Source: three-view drawing plus pictorial views. Frame: mm from the lowest corner of the part. A direction names the side the tool comes from. Give positions to 0.01 mm unless a question says otherwise; leave off trailing zeros. Order: outer loops, then holes, each group sorted by start corner. A loop starts at its lowest first (then second) coordinate and runs counter-clockwise, first axis right, second up. Notation, with made-up numbers: M 31,38 L 44,38 A32 ccw 44,74 Z; hole C 51,61.25 d7. An arc over 180 degrees is marked long. One line per item, written item: value. Start each with the question number.
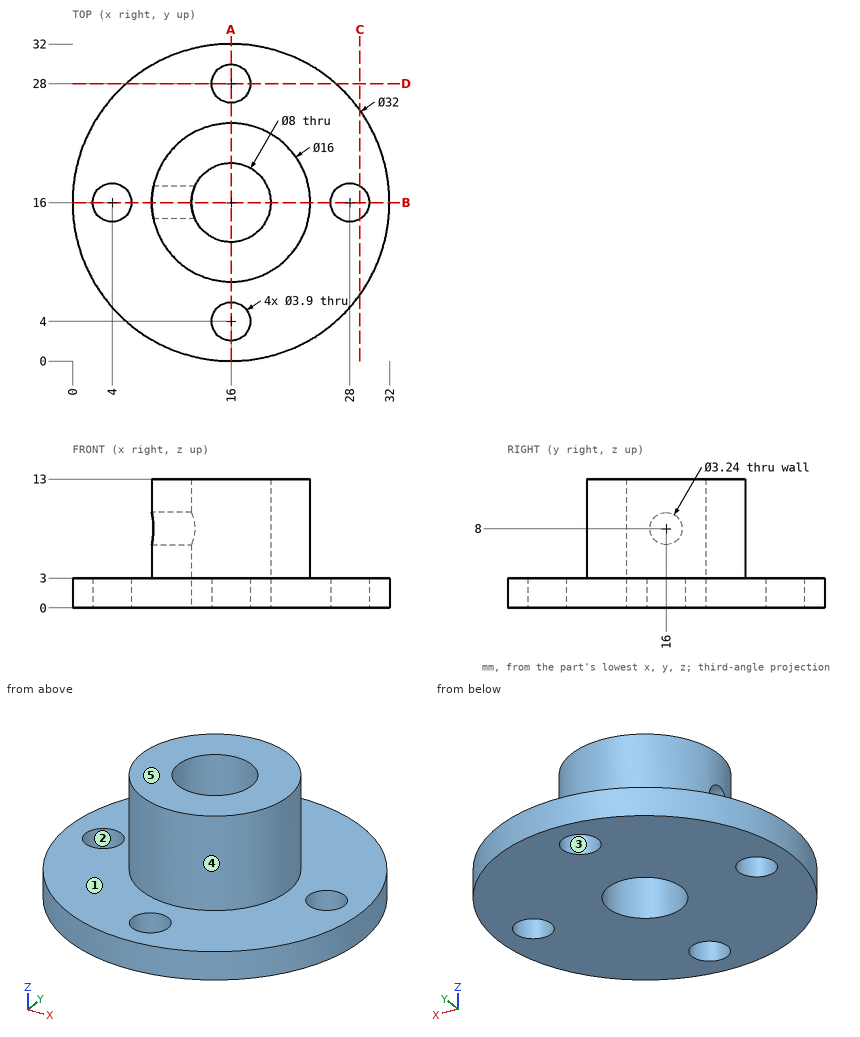
Q1. Section query D-D on y = 28. Return loops of the section in (x, z).
Q2. Section query A-A on x = 16. Return loops of the section in (y, z), and give its area (3 significant figures).
Q3. Mould query, pull axis Y, two halves, no side actions, for the marked faces 3, 4 and 5. Classes: +Y half, -Y half, draft (parallel to the pull), parting line (faces both ways), or undercut.
Q4. Contact query for flat-ended pins moving along their axis: pin 1 (1.9 mm diameter, centred on y = 16, z = 8, fed in from +X); pin 2 (3 mm diameter, centred on x = 14, z = 8.5, fed in from -Y); pin 3 (1.5 mm diameter, centred on x = 28, y = 25.5, fed in from +Z); pin 4 (5 mm diameter, centred on x = 27, z = 11, fed in from -Y) (1 decimal). Output: stop coordinate, or through.
Q5. Ray query, line 1 along Y through (x, z) = (16, 1.6); line 2 along Y through (x, z) = (16, 7); line 3 along Z through (x, y) = (3.5, 9). Return the intervals inside material, ascending. Write a range as [from, to].
Q6. Section query B-B on y = 16. Return loops of the section in (x, z).
Q7. Section query C-C on x = 29. Return loops of the section in (y, z).
Q8. Set-up query: the marked faces 1 and 2. Return all of +Z, -Z, +X, -X, +Y, -Y with unobstructed straight access to the full face (end or side cutting, diameter ignored); none if empty.
Results below:
1. outline: M 5.42,0 L 14.05,0 L 14.05,3 L 5.42,3 Z; M 17.95,0 L 26.58,0 L 26.58,3 L 17.95,3 Z
2. outline: M 0,0 L 2.05,0 L 2.05,3 L 0,3 Z; M 5.95,0 L 12,0 L 12,13 L 8,13 L 8,3 L 5.95,3 Z; M 20,0 L 26.05,0 L 26.05,3 L 24,3 L 24,13 L 20,13 Z; M 29.95,0 L 32,0 L 32,3 L 29.95,3 Z
2. area: 129 mm2
3. face 3: undercut
3. face 4: parting line
3. face 5: draft
4. pin 1: x = 24
4. pin 2: y = 8.02
4. pin 3: z = 3
4. pin 4: through
5. line 1: [0, 2.05], [5.95, 12], [20, 26.05], [29.95, 32]
5. line 2: [8, 12], [20, 24]
5. line 3: [0, 3]
6. outline: M 0,0 L 2.05,0 L 2.05,3 L 0,3 Z; M 5.95,0 L 12,0 L 12,6.38 L 8,6.38 L 8,3 L 5.95,3 Z; M 8,9.62 L 12,9.62 L 12,13 L 8,13 Z; M 20,0 L 26.05,0 L 26.05,3 L 24,3 L 24,13 L 20,13 Z; M 29.95,0 L 32,0 L 32,3 L 29.95,3 Z
7. outline: M 6.67,0 L 14.33,0 L 14.33,3 L 6.67,3 Z; M 17.67,0 L 25.33,0 L 25.33,3 L 17.67,3 Z
8. face 1: +Z
8. face 2: +Z, -Z
